Drawing for the job (mm, zero at the part's lowest x, y, z). Round coordinates to 2 decimals unless told otherwise and drop trailing zeros. Order: outer loops, then holes, each group sorted by start corner. A loop starts at its lowest first (then second) coordinate and runs counter-clockwise, first axis right, second up. Notation, with made-up numbers: (72, 49.25) -> (102, 49.25) arc R21 ccw to (102, 55.25) -> close; hole circle Ø7 at (-20, 52.5). An arc over 180 degrees is marked (long way). Use CSV: the item, a comma, the result in double quotes.
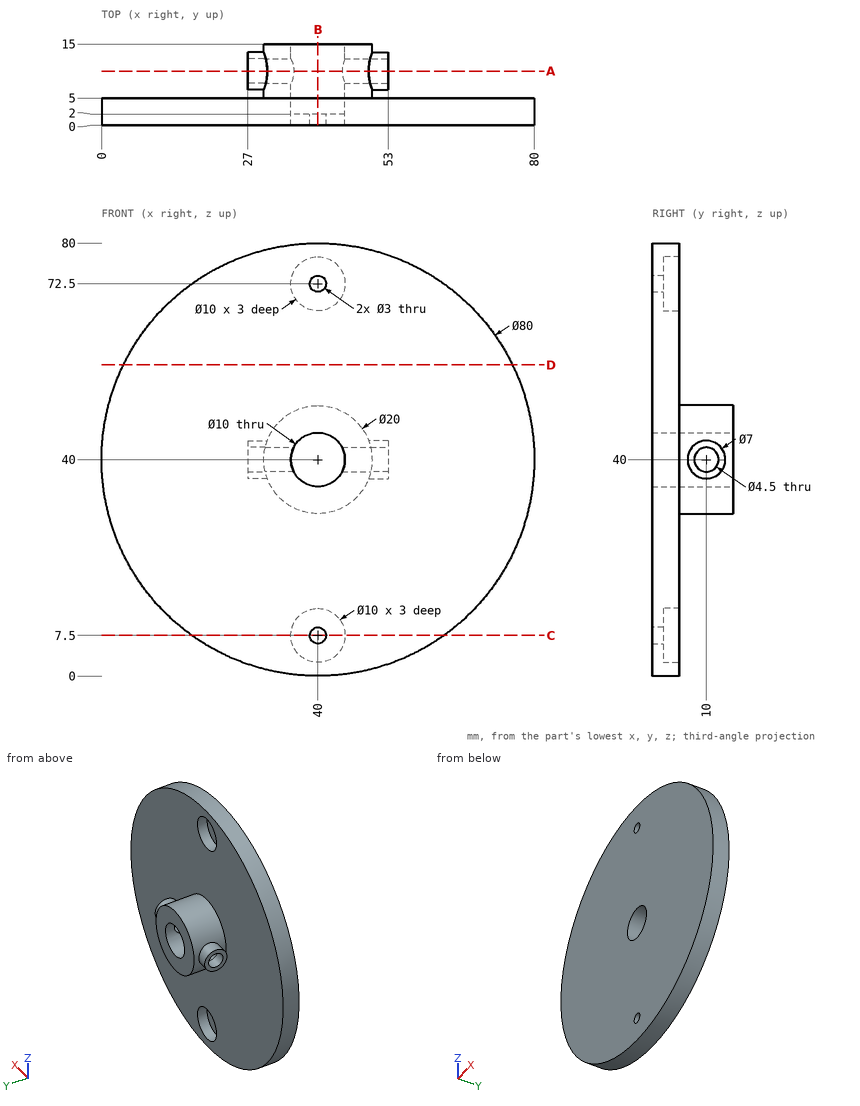
Q1. Cut at A-A (y = 10). Give the cut face in (x, z), plus the area to 3 significant figures.
From the geometry:
outline,"(27, 36.5) -> (30.63, 36.5) arc R10 ccw to (49.37, 36.5) -> (53, 36.5) -> (53, 37.75) -> (44.47, 37.75) arc R5 cw to (35.53, 37.75) -> (27, 37.75) -> close; (27, 42.25) -> (35.53, 42.25) arc R5 cw to (44.47, 42.25) -> (53, 42.25) -> (53, 43.5) -> (49.37, 43.5) arc R10 ccw to (30.63, 43.5) -> (27, 43.5) -> close"
area,"207 mm²"
Q2. Cut at D-D (z = 57.5). Give the cut face in (x, y).
From the geometry:
outline,"(4.03, 0) -> (75.97, 0) -> (75.97, 5) -> (4.03, 5) -> close"
Q3. Probe line 1 along Y through (x, z) = (29.55, 40); line 2 along Y through (x, z) = (67, 52); line 3 along X through (y, z) = (4.15, 72.5). List the from-to ranges inside material, lowest first.
From the geometry:
line 1,"y = 0 to 5, 6.5 to 7.75, 12.25 to 13.5"
line 2,"y = 0 to 5"
line 3,"x = 16.68 to 35, 45 to 63.32"
Q4. Cut at C-C (z = 7.5). Give the cut face in (x, y).
From the geometry:
outline,"(16.68, 0) -> (38.5, 0) -> (38.5, 2) -> (35, 2) -> (35, 5) -> (16.68, 5) -> close; (41.5, 0) -> (63.32, 0) -> (63.32, 5) -> (45, 5) -> (45, 2) -> (41.5, 2) -> close"
Q5. Pin check, flat tips, straight feed: pin 1 (3 mm diameter, centred on y = 3, z = 39.5, fed in from -X); pin 2 (6 mm diameter, centred on y = 10, z = 40, fed in from +X); pin 3 (4 mm diameter, centred on x = 40, z = 72.5, fed in from +Y). Stop position of each tip, or through.
From the geometry:
pin 1,"stops at x = 0"
pin 2,"stops at x = 53"
pin 3,"stops at y = 2"
Q6. Cut at B-B (x = 40). Give the cut face in (y, z).
From the geometry:
outline,"(0, 0) -> (5, 0) -> (5, 2.5) -> (2, 2.5) -> (2, 6) -> (0, 6) -> close; (0, 9) -> (2, 9) -> (2, 12.5) -> (5, 12.5) -> (5, 30) -> (15, 30) -> (15, 35) -> (0, 35) -> close; (0, 45) -> (15, 45) -> (15, 50) -> (5, 50) -> (5, 67.5) -> (2, 67.5) -> (2, 71) -> (0, 71) -> close; (0, 74) -> (2, 74) -> (2, 77.5) -> (5, 77.5) -> (5, 80) -> (0, 80) -> close"
